The listing builds one solid part. Answer for the finished solid, in the listing's coordinates (mm). A direction names the side the tool comes from. Coordinates: 2 decimals unless noted, no trailing zeros. Write each loop counter-clockwise with the first axis right and the second up, starting at its lowest first coordinate (ties: lowest second). Pieces come first, ordered by that corner, then holes.
```python
from build123d import *

# Parameters (mm, degrees)
F1_DEPTH = 20


# Not quite as in the source:
# - a feature names something its author has since deleted; it is built from what else it names


with BuildPart() as f1:
    # F0 (on Top) → F1 (new body)
    with BuildSketch(Plane.XY):
        with BuildLine():
            ThreePointArc((-29.1418942418, 9), (-19.4766119099, 23.471505885), (-3.470733695, 30.3018812554))
            Line((-3.470733695, 30.3018812554), (-3.470733695, 39.8491406133))
            ThreePointArc((-3.470733695, 39.8491406133), (-26.2357325621, 30.1941440834), (-38.9743505398, 9))
            Line((-38.9743505398, 9), (-29.1418942418, 9))
        make_face()
        with BuildLine():
            ThreePointArc((-29.1418942418, -9), (-30.5, 0), (-29.1418942418, 9))
            Line((-29.1418942418, 9), (-38.9743505398, 9))
            ThreePointArc((-38.9743505398, 9), (-40, 0), (-38.9743505398, -9))
            Line((-38.9743505398, -9), (-29.1418942418, -9))
        make_face()
        with BuildLine():
            ThreePointArc((-3.470733695, -30.3018812554), (-19.4766119099, -23.471505885), (-29.1418942418, -9))
            Line((-29.1418942418, -9), (-38.9743505398, -9))
            ThreePointArc((-38.9743505398, -9), (-26.2357325621, -30.1941440834), (-3.470733695, -39.8491406133))
            Line((-3.470733695, -39.8491406133), (-3.470733695, -30.3018812554))
        make_face()
        with BuildLine():
            ThreePointArc((-38.9743505398, -9), (-40, 0), (-38.9743505398, 9))
            Line((-38.9743505398, 9), (-101.2608483434, 9))
            Line((-101.2608483434, 9), (-101.2608483434, -9))
            Line((-101.2608483434, -9), (-38.9743505398, -9))
        make_face()
    extrude(amount=F1_DEPTH)


solid = f1.part
```
(1) For a pull along Z with two mould halves and no side action, classify faces 1 (the flat face through (-49, 0, 0)), 2 (the flat face through (-101.261, 0, 10)), 3 (the flat face through (-49, 0, 20)) as pulls with the +Z half, pulls with the -Z half, needs draft (parallel to the pull), parting line crosses it, or undercut.
(2) Which of the six approach directions +Z, -Z, +X, -X, +Y, -Y give full straight-line access (tool end or side, diameter ignored) to faces 4 (the flat face through (-71, -9, 10)), 5 (the flat face through (-3.471, -35, 10)), 6 (the flat face through (-70, 9, 10))?
(3) Find the intervals of material crossed by probe 1 along Y at (x, z) = (-86, 15.5); probe 2 along Y at (x, z) = (-26, 15); probe 3 along Y at (x, z) = (-18, 18), in increasing order.
(4) Section D-D, the plane x = -32 is taken. Write down the section's boundary in (y, z).
(5) Section B-B, the plane x = -16.5 is taken. Write down the section's boundary in (y, z), plus the area to 3 significant figures.
(6) Section A-A, the plane z = 15.75 is taken. Write down the section's boundary in (x, y), plus the area to 3 significant figures.
(7) Section C-C, the plane y = 5.5 is taken. Write down the section's boundary in (x, z).
(8) Each of these flat-tipped pins is pushed along its axis until it touches: pin 1 (10 mm diameter, centred on x = -18.5, z = 9, fed in from -Y); pin 2 (10 mm diameter, centred on x = -56.5, z = 13.5, fed in from +Y); pin 3 (12 mm diameter, centred on x = -76, z = 10.5, fed in from -Y). Where does it stop, or does it pass through?
Solution:
1. face 1: pulls with the -Z half
1. face 2: needs draft
1. face 3: pulls with the +Z half
2. face 4: +Z, -Z, -X, -Y
2. face 5: +Z, -Z, +X, +Y, -Y
2. face 6: +Z, -Z, -X, +Y
3. probe 1: y = -9 to 9
3. probe 2: y = -30.4 to -15.95, 15.95 to 30.4
3. probe 3: y = -35.72 to -24.62, 24.62 to 35.72
4. outline: (-24, 0) - (24, 0) - (24, 20) - (-24, 20) - close
5. outline: (-36.44, 0) - (-25.65, 0) - (-25.65, 20) - (-36.44, 20) - close; (25.65, 0) - (36.44, 0) - (36.44, 20) - (25.65, 20) - close
5. area: 431 mm2
6. outline: (-101.26, -9) - (-38.97, -9) arc R40 ccw to (-3.47, -39.85) - (-3.47, -30.3) arc R30.5 cw to (-3.47, 30.3) - (-3.47, 39.85) arc R40 ccw to (-38.97, 9) - (-101.26, 9) - close
6. area: 2,090 mm2
7. outline: (-101.26, 0) - (-30, 0) - (-30, 20) - (-101.26, 20) - close
8. pin 1: stops at y = -37.65
8. pin 2: stops at y = 9
8. pin 3: stops at y = -9
